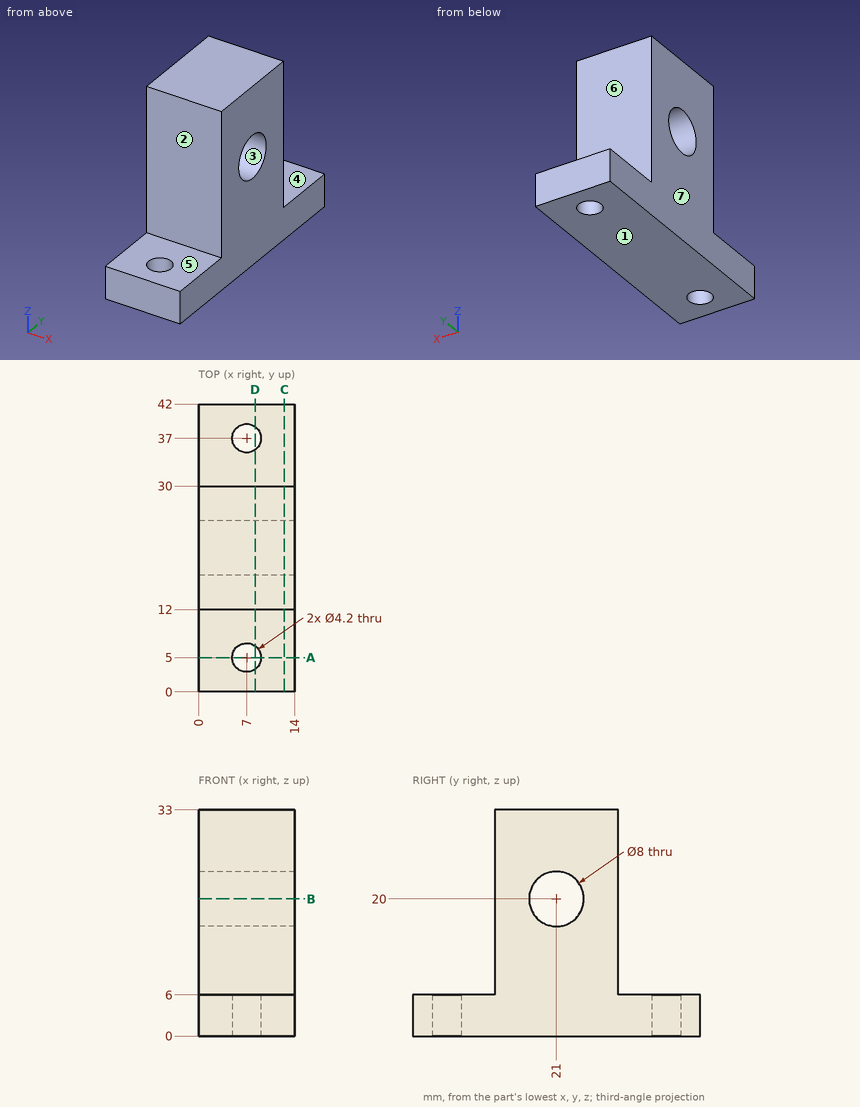
Answer from the drawing. Dimensions are ordinates in mm from the lowest x, y and z of the part. A direction names the side the tool comes from. Coordinates: 2 decimals unless noted, no trailing zeros. Loops run counter-clockwise (first coordinate to the right, second up) from the corner with the lowest first, then second, coordinate; pieces in that order, holes last. Notation, with made-up numbers: (2, 47) - (52, 47) arc R26 ccw to (52, 81) - close; hole circle Ø7 at (82, 50). An arc over 180 degrees is marked (long way). Use a Markdown table: item, result.
Item 1: Find section A-A, the plane y = 5. Determine the outline of the cut face in (x, z).
Evaluation:
| item | result |
|---|---|
| outline | (0, 0) - (4.9, 0) - (4.9, 6) - (0, 6) - close; (9.1, 0) - (14, 0) - (14, 6) - (9.1, 6) - close |
Item 2: Consider probe 1 along Y at (x, z) = (7, 2.7); probe 2 along Z at (x, y) = (5, 21); probe 3 along Z at (x, y) = (3.25, 2). Determine where each line is inside the solid, lowest interval first. Write a range as from..to.
Evaluation:
| item | result |
|---|---|
| probe 1 | y = 0..2.9, 7.1..34.9, 39.1..42 |
| probe 2 | z = 0..16, 24..33 |
| probe 3 | z = 0..6 |
Item 3: The mould has two halves that part along Z. Classify the marked faces 1, 2, 3 and 4: +Z half, -Z half, draft (parallel to the pull), parting line (faces both ways), or undercut.
Evaluation:
| item | result |
|---|---|
| face 1 | -Z half |
| face 2 | draft |
| face 3 | undercut |
| face 4 | +Z half |
Item 4: Find section C-C, the plane x = 12.5. Determine the outline of the cut face in (y, z).
Evaluation:
| item | result |
|---|---|
| outline | (0, 0) - (42, 0) - (42, 6) - (30, 6) - (30, 33) - (12, 33) - (12, 6) - (0, 6) - close; hole circle Ø8 at (21, 20) |
Item 5: For the marked faces 5, 6 and 7, determine the directions among +Z, -Z, +X, -X, +Y, -Y from which every point of the face is accessible in a straight line to the end or side of a thin tool.
Evaluation:
| item | result |
|---|---|
| face 5 | +Z, +X, -X, -Y |
| face 6 | +Z, +X, -X, +Y |
| face 7 | +Z, -Z, -X, +Y, -Y |
Item 6: Find section B-B, the plane z = 20. Determine the outline of the cut face in (x, y), and give its area (3 significant figures).
Evaluation:
| item | result |
|---|---|
| outline | (0, 12) - (14, 12) - (14, 17) - (0, 17) - close; (0, 25) - (14, 25) - (14, 30) - (0, 30) - close |
| area | 140 mm2 |
Item 7: Given pin 1 Ø2 at (x, z) = (5, 16.5) entering from -Y; pin 2 Ø5.5 at (x, y) = (7, 5) entering from +Z, each flat-ended and moving along its own axis, determine where each tip first touches the part or whether it passes through.
Evaluation:
| item | result |
|---|---|
| pin 1 | stops at y = 12 |
| pin 2 | stops at z = 6 |
Item 8: Find section D-D, the plane x = 8.25. Determine the outline of the cut face in (y, z).
Evaluation:
| item | result |
|---|---|
| outline | (0, 0) - (3.31, 0) - (3.31, 6) - (0, 6) - close; (6.69, 0) - (35.31, 0) - (35.31, 6) - (30, 6) - (30, 33) - (12, 33) - (12, 6) - (6.69, 6) - close; (38.69, 0) - (42, 0) - (42, 6) - (38.69, 6) - close; hole circle Ø8 at (21, 20) |
